Part model, mm, in its own coordinate system. A direction names the side the tool comes from. Round coordinates to 2 decimals unless told otherwise and drop trailing zeros. Order: outer loops, then holes, each group sorted by start corner. A loop starts at its lowest first (then second) coordinate and runs counter-clockwise, first axis right, second up. Notation, with made-up numbers: M -6,-17 L 48,-17 A20 cw 48,9 Z; hole C -38.5,31.25 d5. An arc over 180 degrees is marked long. Write each question's results on one line, items separated by ' | '. Start each with the question number.
1. Band-saw the part on A-A, the plane y = 12.5. List the corners of the cut face in (x, z), then the cut area to 3 significant figures.
2. Band-saw the part on B-B, the plane x = -104. List the corners of the cut face in (y, z), then the cut area to 3 significant figures.
3. Probe L1, parallel to X at y = 14.5, z = 5.5; L2, parallel to X at y = 13.5, z = 0.5; L3, parallel to Z at x = -100.5, y = 9.5. List the from-to ranges inside material, lowest first. Write a range as [from, to].
4. Band-saw the part on D-D, the plane x = -98.5. List the corners of the cut face in (y, z), then the cut area to 3 significant figures.
5. Two-plate mould, pull along Y, no slides. Class faces 4 (the face through (-95.17, 9.3, 0.49)), 5 (the face through (-122, 12, 7.408)), 6 (the face through (-111.714, -1.894, 3.652)): +Y half, -Y half, draft (parallel to the pull), parting line (faces both ways), or undercut.
6. Drop flat-ended pins along their axis: pin 1 Ø1 at (x, z) = (-99, 5.5) entering from +Y; pin 2 Ø2 at (x, z) = (-105, 5) entering from +Y; pin 3 Ø3 at (y, z) = (10.5, 1) entering from -X; pin 4 Ø5.5 at (x, y) = (-108.04, 14.64) entering from -Z. Give the stop position or say it passes through.
7. Which spindle directions (+Z, -Z, +X, -X, +Y, -Y) get a long thin tool onto all of the face, cutting with end or side? Do faces 1 (the face through (-114.6, 14.9, 0.5)), 2 (the face through (-102, 11.7, 6.408)), 3 (the face through (-122, 12, 0)). Say none if no direction does.
8. Band-saw the part on C-C, the plane y = 28. List the corners of the cut face in (x, z), then the cut area to 3 significant figures.
```python
from build123d import *

# Parameters (mm, degrees)
SKETCH1_R           = 16.933333333
SKETCH1_R_2         = 4.5625
BOSS_EXTRUDE1_DEPTH = 7.408333333
SKETCH2_R           = 13.933333333
SKETCH2_R_2         = 6.5625
CUT_EXTRUDE1_DEPTH  = 1


with BuildPart() as part:
    # Sketch1 → Boss-Extrude1 (new body)
    with BuildSketch(Plane.XY):
        with Locations((-108.042890629, 14.636479869)):
            Circle(SKETCH1_R)
        with Locations((-108.042890629, 14.636479869)):
            Circle(SKETCH1_R_2, mode=Mode.SUBTRACT)
    extrude(amount=BOSS_EXTRUDE1_DEPTH)

    # Sketch2 → Cut-Extrude1 (cut)
    with BuildSketch(Plane.XY.offset(7.408333333)):
        with Locations((-108.042890629, 14.636479869)):
            Circle(SKETCH2_R)
        with Locations((-108.042890629, 14.636479869)):
            Circle(SKETCH2_R_2, mode=Mode.SUBTRACT)
    cut_extrude1 = extrude(amount=-CUT_EXTRUDE1_DEPTH, mode=Mode.SUBTRACT)

    # Mirror1: Cut-Extrude1 across plane
    add(cut_extrude1.mirror(Plane.XY.offset(3.704166667)), mode=Mode.SUBTRACT)


solid = part.part
```
Solution:
1) outline: M -124.84,0 L -121.81,0 L -121.81,1 L -114.25,1 L -114.25,0 L -112.07,0 L -112.07,7.41 L -114.25,7.41 L -114.25,6.41 L -121.81,6.41 L -121.81,7.41 L -124.84,7.41 Z; M -104.01,0 L -101.84,0 L -101.84,1 L -94.27,1 L -94.27,0 L -91.24,0 L -91.24,7.41 L -94.27,7.41 L -94.27,6.41 L -101.84,6.41 L -101.84,7.41 L -104.01,7.41 Z | area: 159 mm^2
2) outline: M -1.81,0 L 1.3,0 L 1.3,1 L 9.47,1 L 9.47,0 L 12.52,0 L 12.52,7.41 L 9.47,7.41 L 9.47,6.41 L 1.3,6.41 L 1.3,7.41 L -1.81,7.41 Z; M 16.75,0 L 19.81,0 L 19.81,1 L 27.97,1 L 27.97,0 L 31.08,0 L 31.08,7.41 L 27.97,7.41 L 27.97,6.41 L 19.81,6.41 L 19.81,7.41 L 16.75,7.41 Z | area: 180 mm^2
3) L1: [-124.98, -112.6], [-103.48, -91.11] | L2: [-124.94, -121.93], [-114.51, -112.46], [-103.62, -101.58], [-94.16, -91.15] | L3: [1, 6.41]
4) outline: M 0.65,0 L 4.48,0 L 4.48,1 L 24.79,1 L 24.79,0 L 28.62,0 L 28.62,7.41 L 24.79,7.41 L 24.79,6.41 L 4.48,6.41 L 4.48,7.41 L 0.65,7.41 Z | area: 167 mm^2
5) face 4: undercut | face 5: draft | face 6: parting line
6) pin 1: y = 29.26 | pin 2: y = 31.45 | pin 3: x = -124.77 | pin 4: through
7) face 1: -Z | face 2: +Z | face 3: -Z, +X, -X, +Y, -Y
8) outline: M -118.44,0 L -111.99,0 L -111.99,1 L -104.1,1 L -104.1,0 L -97.64,0 L -97.64,7.41 L -104.1,7.41 L -104.1,6.41 L -111.99,6.41 L -111.99,7.41 L -118.44,7.41 Z | area: 138 mm^2
